Input: part model. Units: mm. Frame: model coordinates. Face numbers are marked on the shaded views. A direction names the side the tool comes from. Give positions to 0.01 mm unless a question says otherwise; leave off trailing zeros. Loops run counter-clockwise (first coordinate to the right, second up) from the corner with the lowest first, then second, coordinate; pieces in that order, holes last. Notation, with made-up numbers: (67, 60.5) -> (101, 60.5) arc R33 ccw to (101, 94.5) -> close; hole circle Ø4 at (-11.75, 37.25). An arc over 180 degrees is marked (long way). Answer as a JSON object with one key per item and string values.
```python
from build123d import *

# Parameters (mm, degrees)
SKETCH1_R           = 19.05
SKETCH1_R_2         = 11.1125
BOSS_EXTRUDE1_DEPTH = 76.2
SKETCH2_R           = 16.66875
SKETCH2_R_2         = 11.1125
BOSS_EXTRUDE2_DEPTH = 31.75


with BuildPart() as part:
    # Sketch1 → Boss-Extrude1 (new body)
    with BuildSketch(Plane(origin=(0, 0, 0), x_dir=(1, 0, 0), z_dir=(0, 1, 0))):
        Circle(SKETCH1_R)
        Circle(SKETCH1_R_2, mode=Mode.SUBTRACT)
    extrude(amount=BOSS_EXTRUDE1_DEPTH)

    # Sketch2 → Boss-Extrude2 (add)
    with BuildSketch(Plane(origin=(0, 76.2, 0), x_dir=(1, 0, 0), z_dir=(0, 1, 0))):
        Circle(SKETCH2_R)
        Circle(SKETCH2_R_2, mode=Mode.SUBTRACT)
    extrude(amount=BOSS_EXTRUDE2_DEPTH)

    # Sketch3 → Cut-Revolve1 (revolve, cut)
    with BuildSketch(Plane(origin=(0, 0, 0), x_dir=(0, 0, -1), z_dir=(1, 0, 0))):
        Polygon((16.66875, 107.95), (16.66875, 100.57660721), (11.1125, 107.95), align=None)
    revolve(axis=Axis((0, 107.95, 0), (0, 1, 0)), mode=Mode.SUBTRACT)

    # Sketch8 → Cut-Revolve4 (revolve, cut)
    with BuildSketch(Plane.XY):
        with BuildLine():
            Line((0, 0), (-3.369464108, 0))
            ThreePointArc((-3.369464108, 0), (-11.368836441, 0.801722978), (-19.05, 3.175))
            Line((-19.05, 3.175), (-19.05, -4.469484217))
            Line((-19.05, -4.469484217), (0, -4.469484217))
            Line((0, -4.469484217), (0, 0))
        make_face()
    revolve(axis=Axis((0, 0, 0), (0, 1, 0)), mode=Mode.SUBTRACT)


solid = part.part
```
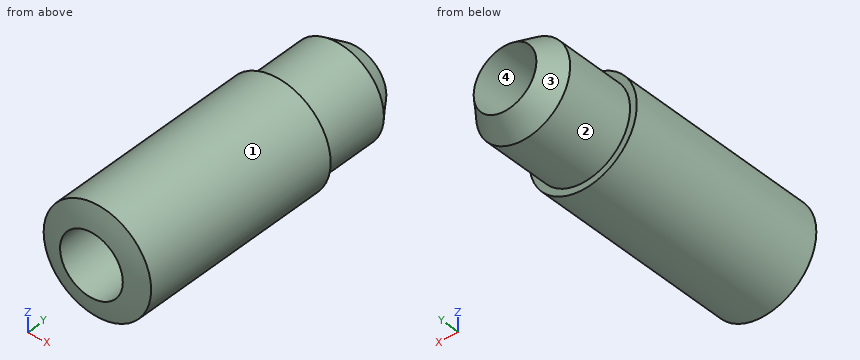
Q1. Draft query along Z for the marked faces 3 and 4. Return one class per face: +Z half, -Z half, draft (parallel to the pull), parting line (faces both ways), or undercut.
Evaluation:
{"face 3": "parting line", "face 4": "undercut"}
Q2. Pin query (flat end, axial travel): pin 1 (4 mm diameter, centred on x = -7, y = 39, fed in from -Z); pin 2 (4 mm diameter, centred on x = 7.5, z = 13, fed in from -Y); pin 3 (5 mm diameter, centred on x = -5.5, y = 18.5, fed in from -Z). Return the tip coordinate at first contact, or that it passes through.
Evaluation:
{"pin 1": "stops at z = -18.38", "pin 2": "stops at y = 1.17", "pin 3": "stops at z = -18.81"}
Q3. Access query for the marked faces 1 and 2. Directions: +Z, -Z, +X, -X, +Y, -Y. A direction counts if a zero-diameter tool reaches every point of the face in a straight line with its end or side. Return the directions, or none.
Evaluation:
{"face 1": "+Y, -Y", "face 2": "+Y"}
Q4. Section B-B, the plane y = 80. Return the cut outline in (x, z) (1 decimal).
Evaluation:
{"outline": "circle Ø33.3 at (0, 0); hole circle Ø22.2 at (0, 0)"}
Q5. Ray query, line 1 along Z through (x, y) = (0, 53); line 2 along Z through (x, y) = (-1, 102.5). Return the intervals inside material, ascending.
Evaluation:
{"line 1": "z = -19.05 to -11.11, 11.11 to 19.05", "line 2": "z = -15.19 to -11.07, 11.07 to 15.19"}
